Geometry check sheet. Reference: the model listing, model coordinates, mm. A direction names the side the tool comes from. Round coordinates to 2 decimals unless told otherwise and drop trailing zeros. Order: outer loops, then holes, each group sorted by start corner. A loop starts at its lowest first (then second) coordinate and runs counter-clockwise, first axis right, second up. Notation, with made-up numbers: M 9.25,-9 L 49.25,-9 A18 ccw 49.25,25 Z; hole C 38.5,-10 d11. An arc over 180 degrees is marked long. Answer as a JSON object with one key per item and string values. Group by question number.
```python
from build123d import *

# Parameters (mm, degrees)
CUT_EXTRUDE1_DEPTH      = 7
CUT_EXTRUDE2_DEPTH      = 0.5
CUT_EXTRUDE2_DEPTH_BACK = 7
SKETCH5_R               = 1.5
SKETCH6_R               = 1
CUT_EXTRUDE3_DEPTH      = 15.204074326


with BuildPart() as part:
    # Sketch3 → Revolve1 (revolve)
    with BuildSketch(Plane(origin=(0, 0, 0), x_dir=(0, 0, -1), z_dir=(1, 0, 0)), mode=Mode.PRIVATE) as revolve1_sk:
        with BuildLine():
            Line((0, 0), (7, 0))
            Line((7, 0), (7, 5.528405338))
            ThreePointArc((7, 5.528405338), (6.72879079, 5.972989159), (6.209380903, 5.935272074))
            Line((6.209380903, 5.935272074), (3.790619097, 4.207585069))
            ThreePointArc((3.790619097, 4.207585069), (3.5, 4.114451805), (3.209380903, 4.207585069))
            Line((3.209380903, 4.207585069), (0.790619097, 5.935272074))
            ThreePointArc((0.790619097, 5.935272074), (0.27120921, 5.972989159), (0, 5.528405338))
            Line((0, 5.528405338), (0, 0))
        make_face()
    revolve(revolve1_sk.sketch.rotate(Axis((0, 0, 0), (0, 0, -1)), 90), axis=Axis((0, 0, 0), (0, 0, -1)))

    # Sketch4 → Cut-Extrude1 (cut)
    with BuildSketch(Plane.XY):
        with BuildLine():
            Line((-1.29614814, 1.1), (1.29614814, 1.1))
            ThreePointArc((1.29614814, 1.1), (0, -1.7), (-1.29614814, 1.1))
        make_face()
    extrude(amount=-CUT_EXTRUDE1_DEPTH, mode=Mode.SUBTRACT)

    # Sketch5 → Cut-Extrude2 (cut, two sides: drawn at the far end of the back side and taken through both)
    with BuildSketch(Plane.XZ.offset(-1.1).offset(-CUT_EXTRUDE2_DEPTH_BACK)):
        with Locations(Location((0, -3.5, 0), (0, 0, 149.779954189))):
            Circle(SKETCH5_R)
    extrude(amount=CUT_EXTRUDE2_DEPTH + CUT_EXTRUDE2_DEPTH_BACK, mode=Mode.SUBTRACT)

    # Sketch6 → Cut-Extrude3 (cut, through all)
    with BuildSketch(Plane(origin=(-3.719471212, 3.156597774, -2.27027027), x_dir=(-0.4225088351551143, 0.39998024596887827, 0.8133277857361964), z_dir=(-0.620423014647787, 0.5265334225455343, -0.5812381937190964))):
        with Locations(Location((-0.01464323, -2.617517623, 0), (0, 0, 358.190705297))):
            Circle(SKETCH6_R)
    extrude(amount=-CUT_EXTRUDE3_DEPTH, mode=Mode.SUBTRACT)


solid = part.part
```
1) Sectioned sample at D-D (z = -4.5). Record the boundary of the cut face in (x, y).
2) Thickness scan on line 1 along Z through (x, y) = (0, 3.15); line 2 along X through (y, z) = (1.75, -4.5); line 3 along Y through (x, z) = (1.25, -6.5). Record the ranges inside material, lowest first. Write a range as [from, to].
3) Sectioned sample at B-B (y = -0.25). Count the separate pieces of the cut face and the enclosed holes in it, then the cut area to 3 significant figures.
4) Go/stop test with flat-tipped pins: P1, Ø4, axis at x = 0, z = -3.5, coming from the -Y side; P2, Ø3, axis at x = 4.5, z = -4.5, coming from the -Y side; P3, Ø2, axis at x = 0, z = -2, coming from the -Y side. Record where each tip stops, or that it passes through.
5) Release check for a two-part mould opening along X. For faces 1 (the conical face through (-0.58, -4.45, -4.18)), 2 (the flat face through (2, 0, 0)), 3 (the flat face through (0, 1.1, -6)) record: +X half, -X half, draft (parallel to the pull), parting line (faces both ways), or undercut.
6) Sectioned sample at A-A (x = 0). Record the boundary of the cut face in (y, z), then the cut area to 3 significant figures.
7) Sectioned sample at C-C (z = -3). Record the boundary of the cut face in (x, y), then the cut area to 3 significant figures.
8) Set-up check for faces 4 (the flat face through (0, 1.1, -1)), 5 (the conical face through (2.32, -3.64, -3.06)), 6 (the flat face through (1.31, -1.31, -7)), 7 (the cylindrical face through (-1.33, 2.97, -4.19)): record each of +Z, -Z, +X, -X, +Y, -Y from which the full face is reachable in a straight line by a thin tool's end or side.
Final values:
{
 "1": {"outline": "M -1.3,1.1 L -1.12,1.1 L -1.12,4.58 A4.71 ccw long 1.12,4.58 L 1.12,1.1 L 1.3,1.1 A1.7 cw long Z"},
 "2": {"line 1": "z = [-7, -5], [-2, 0]", "line 2": "x = [-4.38, -1.12], [1.12, 4.38]", "line 3": "y = [-5.9, -1.15], [1.1, 5.9]"},
 "3": {"separate pieces": "3", "enclosed holes": "0", "area": "44.5 mm^2"},
 "4": {"P1": "stops at y = -5.43", "P2": "stops at y = -4.26", "P3": "stops at y = -5.79"},
 "5": {"face 1": "parting line", "face 2": "draft", "face 3": "undercut"},
 "6": {"outline": "M -5.94,-6.21 A0.5 ccw -5.53,-7 L -1.7,-7 L -1.7,0 L -5.53,0 A0.5 ccw -5.94,-0.79 L -4.21,-3.21 A0.5 cw -4.21,-3.79 Z; M 1.1,-7 L 5.53,-7 A0.5 ccw 5.94,-6.21 L 5.07,-5 L 1.1,-5 Z; M 1.1,-2 L 5.07,-2 L 5.94,-0.79 A0.5 ccw 5.53,0 L 1.1,0 Z", "area": "42.8 mm^2"},
 "7": {"outline": "M -1.41,0.94 L -1.41,4.12 A4.36 ccw long 1.41,4.12 L 1.41,0.94 A1.7 cw long Z", "area": "42.6 mm^2"},
 "8": {"face 4": "+Z, -Z", "face 5": "none", "face 6": "-Z, +X, -X, +Y, -Y", "face 7": "+Y"}
}
